Can you work these out from the model? Positions are in its coordinate system, mm. A direction names the side the tool comes from. Give positions to 0.01 mm unless a question says otherwise; leave off trailing zeros. Order: outer loops, then holes, each group sorted by start corner. A loop starts at its lowest first (then second) coordinate and runs counter-clockwise, first axis right, second up. Notation, with made-up numbers: (12.25, 7) -> (59.25, 7) arc R28 ccw to (59.25, 31) -> close; hole circle Ø1 at (87.5, 60.25). An arc over 180 degrees is marked (long way). Answer as a JSON object with one key per item and string values.
```python
from build123d import *

# Parameters (mm, degrees)
F0_W     = 25.4
F0_H     = 13.1786093116
F1_DEPTH = 63.5


with BuildPart() as f1:
    # F0 (on Front) → F1 (new body, symmetric)
    with BuildSketch(Plane.XZ):
        Polygon((-40.1599369943, -9.525), (40.1599369943, -9.525), (40.1599369943, 9.525), (31.7779369652, 9.525), (-40.1599369943, 9.525), align=None)
        with BuildLine():
            Line((31.7779369652, 9.525), (40.1599369943, 9.525))
            Line((40.1599369943, 9.525), (40.1599369943, 68.4023214343))
            ThreePointArc((40.1599369943, 68.4023214343), (45.0018921637, 75.3878619554), (53.2423900817, 73.3054354144))
            Line((53.2423900817, 73.3054354144), (54.1008195247, 73.3054354144))
            Line((54.1008195247, 73.3054354144), (54.1008195247, 82.8580701694))
            ThreePointArc((54.1008195247, 82.8580701694), (39.0089250876, 81.6996873131), (31.7779369652, 68.4023214343))
            Line((31.7779369652, 68.4023214343), (31.7779369652, 9.525))
        make_face()
        with BuildLine():
            add(Edge.make_bspline(
                [(-40.1599369943, 9.525), (8.3736795932, 33.7357372046), (-11.0195567831, 69.6132257581), (31.7779369652, 68.4023214343)],
                knots=[0, 0, 0, 0, 92.960188732, 92.960188732, 92.960188732, 92.960188732], degree=3))
            Line((-40.1599369943, 9.525), (31.7779369652, 9.525))
            Line((31.7779369652, 9.525), (31.7779369652, 68.4023214343))
        make_face()
        with BuildLine():
            ThreePointArc((56.2499082782, 81.6874354435), (55.198002297, 82.3143130986), (54.1008195247, 82.8580701694))
            Line((54.1008195247, 82.8580701694), (54.1008195247, 73.3054354144))
            Line((54.1008195247, 73.3054354144), (79.5008195247, 73.3054354144))
            Line((79.5008195247, 73.3054354144), (79.5008195247, 81.6874354435))
            Line((79.5008195247, 81.6874354435), (56.2499082782, 81.6874354435))
        make_face()
        with BuildLine():
            Line((54.1008195247, 86.484044726), (54.1008195247, 82.8580701694))
            ThreePointArc((54.1008195247, 82.8580701694), (55.198002297, 82.3143130986), (56.2499082782, 81.6874354435))
            Line((56.2499082782, 81.6874354435), (79.5008195247, 81.6874354435))
            Line((79.5008195247, 81.6874354435), (79.5008195247, 86.484044726))
            Line((79.5008195247, 86.484044726), (54.1008195247, 86.484044726))
        make_face()
        with Locations((66.8008195247, 66.7161307586)):
            Rectangle(F0_W, F0_H)
        Polygon((79.5008195247, 81.6874354435), (79.5008195247, 73.3054354144), (79.5008195247, 60.1268261029), (104.9008195247, 60.1268261029), (104.9008195247, 86.484044726), (79.5008195247, 86.484044726), align=None)
    extrude(amount=F1_DEPTH, both=True)


solid = f1.part
```
1. For faces 5 (the face through (54.101, -1, 67)), 6 (the face through (-1, -1, -9.525)), 7 (the face through (79, -1, 60.127)), which set-ups out of +Z, -Z, +X, -X, +Y, -Y let a thin tool reach every point of the face, with its end or its side?
Worked answers:
{"face 5": "-Z, +Y, -Y", "face 6": "-Z, +X, -X, +Y, -Y", "face 7": "-Z, +X, +Y, -Y"}
2. If we mould it in two halves opening along X, with no side actions, what happens to faces 1 (the face through (-40.16, -1, 0)), 2 (the face through (104.901, -1, 73)), 3 (the face through (39.2, -0.89, 81.82)), 4 (the face through (80, -1, 86.484))? For each: +X half, -X half, draft (parallel to the pull), parting line (faces both ways), or undercut.
Worked answers:
{"face 1": "-X half", "face 2": "+X half", "face 3": "undercut", "face 4": "draft"}
3. If we section it at B-B on x = 89.5: Please give me the cut outline in (y, z).
Worked answers:
{"outline": "(-63.5, 60.13) -> (63.5, 60.13) -> (63.5, 86.48) -> (-63.5, 86.48) -> close"}
4. Please list where these lines run through material, in increasing order: L1, parallel to Z at x = 86, y = -5.5; L2, parallel to X at y = 18, z = 0; L3, parallel to Z at x = 27.5, y = 56 (3 decimals).
Worked answers:
{"L1": "60.13 to 86.48", "L2": "-40.16 to 40.16", "L3": "-9.525 to 68.395"}
5. Will these pins go through, and if not, where does the flat tip stop? pin 1 Ø1 at (x, y) = (76, 36.5) entering from -Z; pin 2 Ø0.7 at (x, y) = (53.5, 26) entering from -Z; pin 3 Ø10.5 at (y, z) = (31, 68) entering from -X.
Worked answers:
{"pin 1": "z = 60.13", "pin 2": "z = 73.31", "pin 3": "x = 8.81"}
6. If we section it at A-A on z = -3: Please give me the cut outline in (x, y), then the cut area to 3 significant figures.
Worked answers:
{"outline": "(-40.16, -63.5) -> (40.16, -63.5) -> (40.16, 63.5) -> (-40.16, 63.5) -> close", "area": "10,200 mm²"}
